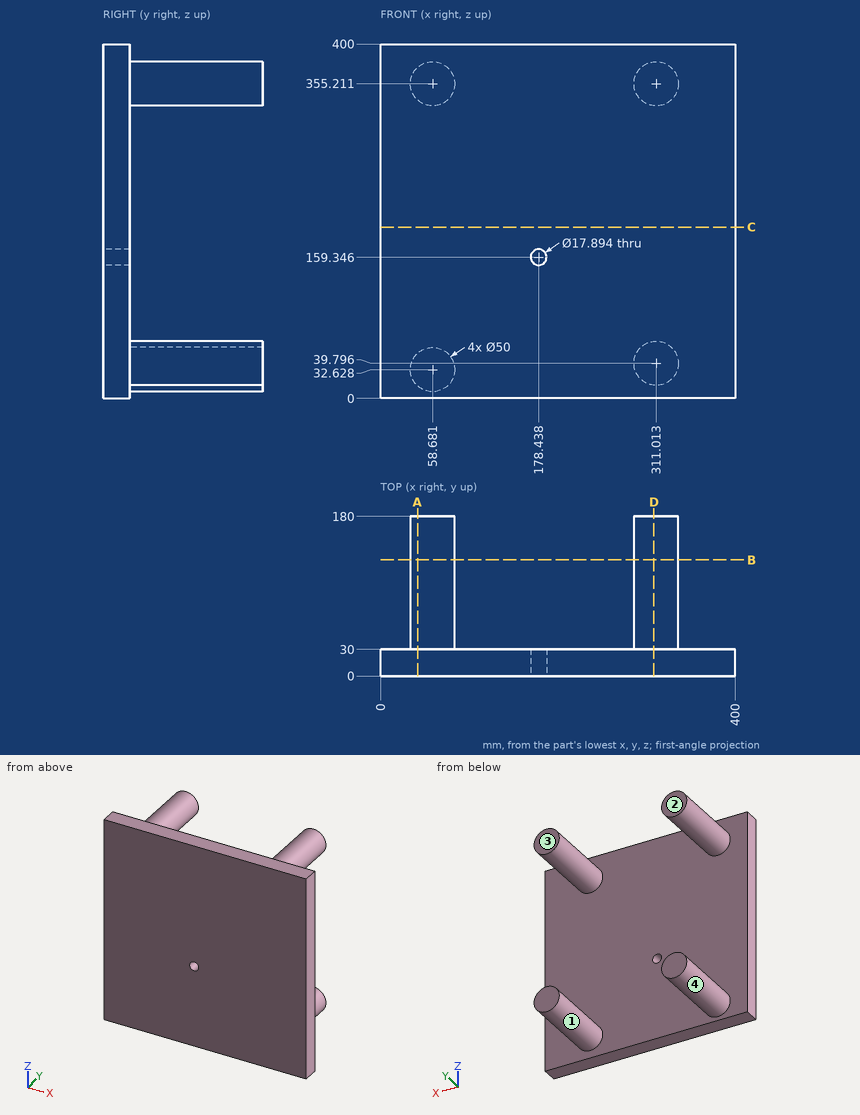
Design review of the part shown in the three views and the two pictorial views. Dimensions are in mm from the part's minimum x, y and z. A direction names the side the tool comes from. Round coordinates to 2 decimals unless told otherwise and drop trailing zeros. Loops run counter-clockwise (first coordinate to the right, second up) from the corner with the lowest first, then second, coordinate; pieces in that order, holes last. Notation, with made-up numbers: M 54,62 L 90,62 A17 ccw 90,74 Z; hole C 35,82 d7. An arc over 180 degrees is marked long. Answer as a JSON object with one key per item and string values.
Item 1: Tool access review of the marked faces 3 and 4: name each direction out of +Z, -Z, +X, -X, +Y, -Y from which nothing blocks a thin tool from reaching the whole face with its end or side.
Check sheet entries:
{"face 3": "+Z, -Z, +X, -X, +Y", "face 4": "+Y"}
Item 2: We need section C-C, the plane z = 193.5. State the section outline as (x, y) points, and give its area (3 significant figures).
Check sheet entries:
{"outline": "M 0,0 L 400,0 L 400,30 L 0,30 Z", "area": "12,000 mm2"}
Item 3: For line 1 along Z through (x, y) = (319, 82) (1 decimal); line 2 along Y through (x, z) = (134, 287.5); line 3 along X through (y, z) = (97, 38.5), list the stretches that pass through material, from the lowest coordinate up.
Check sheet entries:
{"line 1": "16.1 to 63.5, 331.5 to 378.9", "line 2": "0 to 30", "line 3": "34.38 to 82.98, 286.05 to 335.98"}
Item 4: We need section D-D, the plane x = 308.5. State the section outline as (y, z) points (1 decimal), and give its area (3 significant figures).
Check sheet entries:
{"outline": "M 0,0 L 30,0 L 30,14.9 L 180,14.9 L 180,64.7 L 30,64.7 L 30,330.3 L 180,330.3 L 180,380.1 L 30,380.1 L 30,400 L 0,400 Z", "area": "26,900 mm2"}
Item 5: We need section A-A, the plane x = 42. State the section outline as (y, z) points, and give its area (3 significant figures).
Check sheet entries:
{"outline": "M 0,0 L 30,0 L 30,14.01 L 180,14.01 L 180,51.25 L 30,51.25 L 30,336.59 L 180,336.59 L 180,373.83 L 30,373.83 L 30,400 L 0,400 Z", "area": "23,200 mm2"}
Item 6: Clearance check with flat-ended pins moving along their axes: P1, Ø1.5, axis at y = 50.5, z = 342.5, coming from the +X side (1 decimal); P2, Ø3, axis at x = 158.5, z = 272.5, coming from the +Y side; P3, Ø8, axis at x = 336, y = 125, coming from the -Z side. State where each tip first meets the part, or that it passes through.
Check sheet entries:
{"P1": "x = 333", "P2": "y = 30", "P3": "z = 26.21"}
Item 7: We need section B-B, the plane y = 131. State the section outline as (x, z) points, and give its area (3 significant figures).
Check sheet entries:
{"outline": "C 58.68,32.63 d50; C 58.68,355.21 d50; C 311.01,39.8 d50; C 311.01,355.21 d50", "area": "7,850 mm2"}
Item 8: The part is to be moulded in two halves that separate along X. For the marked faces 1 and 2, say which applies: +X half, -X half, draft (parallel to the pull), parting line (faces both ways), or undercut.
Check sheet entries:
{"face 1": "undercut", "face 2": "draft"}
